Can you work these out from the drawing? Everything is in mm from the part's minimum corner. A direction names the side the tool comes from. Coordinates: 2 decimals unless noted, no trailing zeros. Write each loop counter-clockwise with the first axis right and the second up, starting at its lowest first coordinate (ties: lowest second). Pieces come first, ordered by that corner, then holes. Notation, with made-up numbers: (56.25, 43.5) -> (83.25, 43.5) arc R25 ccw to (83.25, 61.5) -> close; hole circle Ø5 at (2.25, -8). An arc over 180 degrees is marked (long way). Answer as CSV lines item,"result". Start each with the question number.
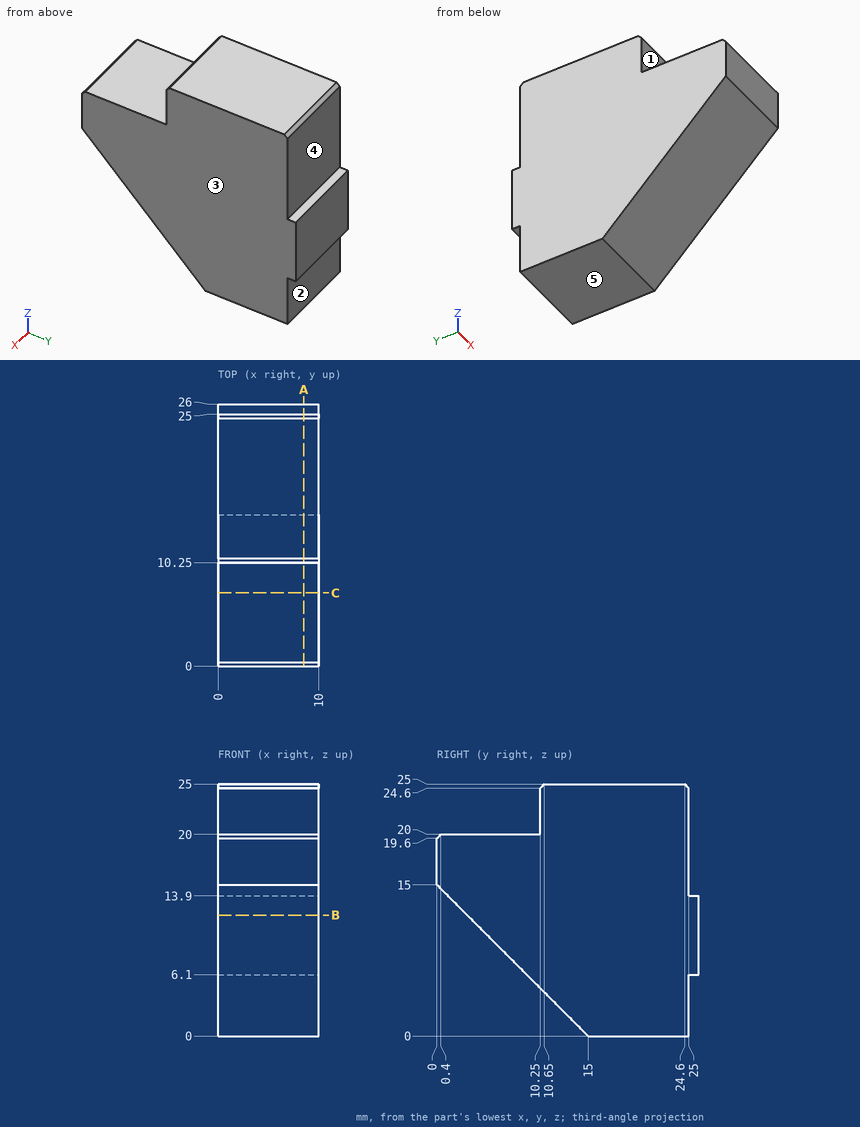
Q1. Imagine slicing it at B-B (z = 12). Write out the boundary of the cut face in (x, y), then the cut area to 3 significant figures.
Q2. I need wall thicknesses on L1, parallel to Y at x = 2.5, z = 22.5; L2, parallel to Y at x = 5.5, z = 16; L3, parallel to Z at x = 5.75, y = 12.5. Which ranges of each line are inside material? Lowest first, please.
Q3. For pin 1 (12 mm diameter, centred on y = 18, z = 17.5, fed in from -X); pin 2 (5 mm diameter, centred on x = 2.5, y = 7, fed in from -Z); pin 3 (1.5 mm diameter, centred on x = 5.5, z = 4.5, fed in from -Y); pin 4 (2.5 mm diameter, centred on x = 5.5, z = 23.5, fed in from -Y), each with a flat end and sliding along its axis, tell me the tip position at first contact or that it passes through.
Q4. Which directions (+Z, -Z, +X, -X, +Y, -Y) give clear straight access to the entire face, cutting with the end or side of a thin tool? Please do the marked faces 1, 2, 3, 4 and 5.
Q5. Imagine slicing it at C-C (y = 7.25). Write out the boundary of the cut face in (x, z), then the cut area to 4 significant figures.
Q6. Imagine slicing it at A-A (x = 8.5). Write out the boundary of the cut face in (y, z), then the cut area to 3 significant figures.
Entries:
1,outline,"(0, 3) -> (10, 3) -> (10, 26) -> (0, 26) -> close"
1,area,"230 mm2"
2,L1,"10.25 to 25"
2,L2,"0 to 25"
2,L3,"2.5 to 25"
3,pin 1,"x = 0"
3,pin 2,"z = 5.5"
3,pin 3,"y = 9.75"
3,pin 4,"y = 10.25"
4,face 1,"+Z, +X, -X, -Y"
4,face 2,"-Z, +X, -X, +Y"
4,face 3,"+Z, -Z, +X, +Y, -Y"
4,face 4,"+Z, +X, -X, +Y"
4,face 5,"-Z, +X, -X, +Y, -Y"
5,outline,"(0, 7.75) -> (10, 7.75) -> (10, 20) -> (0, 20) -> close"
5,area,"122.5 mm2"
6,outline,"(0, 15) -> (15, 0) -> (25, 0) -> (25, 6.1) -> (26, 6.1) -> (26, 13.9) -> (25, 13.9) -> (25, 24.6) -> (24.6, 25) -> (10.65, 25) -> (10.25, 24.6) -> (10.25, 20) -> (0.4, 20) -> (0, 19.6) -> close"
6,area,"469 mm2"
